Verification items for the finished model (mm, model axes). A direction names the side the tool comes from. Give positions to 0.01 mm unless a question says otherwise; leave off trailing zeros. Order: outer loops, then holes, each group sorted by start corner. A loop starts at its lowest first (then second) coordinate and runs counter-clockwise, first axis right, second up. Notation, with made-up numbers: (83.25, -33) - (115.25, -33) arc R14 cw to (115.25, -10) - close; hole circle Ø11 at (16, -27.5). An arc over 180 degrees is marked (long way). Answer as a JSON object with one key per item and string values. Group by question number.
(1) Depth check by flat-ended pin: pin 1 Ø1 at (x, y) = (4, 8) entering from +Z; pin 2 Ø2 at (x, y) = (2, 7) entering from -Z; pin 3 Ø1 at (y, z) = (3.5, -16) entering from +X; pin 4 Ø3 at (y, z) = (5, 18.2) entering from -X. Enter the tip coordinate at first touch or a pass-through.
(2) Mould release check, pull along Z, two halves, no side actions. Record for faces 4 (the face through (0, 5, 10.2)), 5 (the face through (4, 5, -14.2)), 6 (the face through (4, 0, 0)): +Z half, -Z half, draft (parallel to the pull), parting line (faces both ways), or undercut.
(3) Access from +Z, -Z, +X, -X, +Y, -Y to the whole of each face (thin tool, end or side, straight path). Record for faces 1 (the face through (0.25, 2.7, 19.1)), 2 (the face through (0.25, 2.7, -19.1)), 3 (the face through (0, 5, -10.2)).
(4) Thickness scan on line 1 (Z direction, x = -1.5, y = 8.5); line 2 (Z direction, x = -2.25, y = 5.75); line 3 (Y direction, x = -0.55, z = -18.2). Record the ranges inside material, lowest first.
(5) Section check B-B (z = 18.2). Record the boundary of the cut face in (x, y), then the cut area to 3 significant figures.
(6) Section check C-C (x = 2.5). Record the boundary of the cut face in (y, z).
(7) Section check A-A (x = -2.75). Record the boundary of the cut face in (y, z).
(8) Section check D-D (y = 5). Record the boundary of the cut face in (x, z), then the cut area to 3 significant figures.
Autodesk Inventor part; units mm, degrees
ref_plane "YZ Plane" through (0, 0, 0) normal (1, 0, 0) x (0, 1, 0)
ref_plane "XZ Plane" through (0, 0, 0) normal (0, 1, 0) x (-1, 0, 0)
ref_plane "XY Plane" through (0, 0, 0) normal (0, 0, 1) x (1, 0, 0)
sketch "Sketch1" plane through (0, 0, 0) normal (0, 1, 0) x (-1, 0, 0)
  line L0 (-3.75, 10.2) -> (3.75, 10.2)
  line L1 (3.75, -10.2) -> (-3.75, -10.2)
  line L2 (-3.75, -10.2) -> (-3.75, 10.2)
  line L3 (-3.75, 10.2) -> (3.75, -10.2) construction
  line L4 (3.75, 10.2) -> (-3.75, -10.2) construction
  line L5 (3.75, 10.2) -> (3.75, 22.2)
  line L6 (-3.75, 0) -> (6.7195, 0) construction
  line L7 (3.75, -10.2) -> (3.75, -22.2)
  line L8 (3.75, 22.2) -> (-0.25, 22.2)
  line L9 (-0.25, 22.2) -> (-0.25, 14.2)
  line L10 (-0.25, 14.2) -> (-7.75, 14.2)
  line L11 (3.75, -22.2) -> (-0.25, -22.2)
  line L12 (-0.25, -22.2) -> (-0.25, -14.2)
  line L13 (-0.25, -14.2) -> (-7.75, -14.2)
  line L14 (-7.75, 14.2) -> (-7.75, -14.2)
  point P0 (0, 0)
  dimension "d0" = 7.5
  dimension "d1" = 20.4
  dimension "d2" = 12
  dimension "d3" = 7.5
  dimension "d5" = 4
  dimension "d6" = 8
  dimension "d7" = 7.5
extrude "Extrusion1" add sketch "Sketch1" along normal blind 10
sketch "Sketch2" plane through (0.25, 0, 22.2) normal (1, 0, 0) x (0, 0, -1)
  line L0 (22.2, 0) -> (22.2, 12.2527) construction
  line L1 (0, 0) -> (0, 10) construction
  line L2 (8, 0) -> (36.4, 0) construction
  line L3 (0, 10) -> (8, 0) construction
  circle A0 centre (4, 5) radius 2.3
  circle A1 centre (40.4, 5) radius 2.3
  dimension "d10" = 4.6
extrude "Extrusion2" cut sketch "Sketch2" against normal through all
properties part number "3d_print_actuator_mount"
Solutions:
{
 "1": {"pin 1": "stops at z = 14.2", "pin 2": "stops at z = -14.2", "pin 3": "stops at x = 0.25", "pin 4": "passes through"},
 "2": {"face 4": "undercut", "face 5": "-Z half", "face 6": "draft"},
 "3": {"face 1": "+Z, +X, +Y, -Y", "face 2": "-Z, +X, +Y, -Y", "face 3": "-X, +Y, -Y"},
 "4": {"line 1": "z = -22.2 to -10.2, 10.2 to 22.2", "line 2": "z = -22.2 to -20.37, -16.03 to -10.2, 10.2 to 16.03, 20.37 to 22.2", "line 3": "y = 0 to 2.7, 7.3 to 10"},
 "5": {"outline": "(-3.75, 0) - (0.25, 0) - (0.25, 2.7) - (-3.75, 2.7) - close; (-3.75, 7.3) - (0.25, 7.3) - (0.25, 10) - (-3.75, 10) - close", "area": "21.6 mm2"},
 "6": {"outline": "(0, -14.2) - (10, -14.2) - (10, -10.2) - (0, -10.2) - close; (0, 10.2) - (10, 10.2) - (10, 14.2) - (0, 14.2) - close"},
 "7": {"outline": "(0, -22.2) - (10, -22.2) - (10, -10.2) - (0, -10.2) - close; (0, 10.2) - (10, 10.2) - (10, 22.2) - (0, 22.2) - close; hole circle Ø4.6 at (5, -18.2); hole circle Ø4.6 at (5, 18.2)"},
 "8": {"outline": "(-3.75, -22.2) - (0.25, -22.2) - (0.25, -20.5) - (-3.75, -20.5) - close; (-3.75, -15.9) - (0.25, -15.9) - (0.25, -14.2) - (7.75, -14.2) - (7.75, 14.2) - (0.25, 14.2) - (0.25, 15.9) - (-3.75, 15.9) - (-3.75, 10.2) - (3.75, 10.2) - (3.75, -10.2) - (-3.75, -10.2) - close; (-3.75, 20.5) - (0.25, 20.5) - (0.25, 22.2) - (-3.75, 22.2) - close", "area": "201 mm2"}
}
